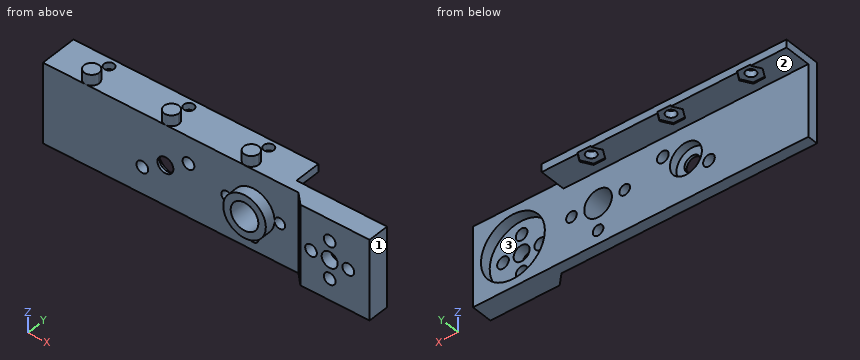
```python
from build123d import *

# Parameters (mm, degrees)
SKETCH_1_W          = 63
SKETCH_1_H          = 15
SKETCH_1_R          = 1.1
SKETCH_1_R_2        = 1
SKETCH_1_R_3        = 1.5
SKETCH_1_R_4        = 2.6
EXTRUDE_1_DEPTH     = 2
EXTRUDE_2_DEPTH     = 2
SKETCH_4_R          = 3
CUT_EXTRUDE_1_DEPTH = 1.5
SKETCH_5_W          = 46
SKETCH_5_H          = 1.5
EXTRUDE_3_DEPTH     = 5
SKETCH_2_3_R        = 0.95
CUT_EXTRUDE_2_DEPTH = 6
CUT_EXTRUDE_START   = -0.25
SKETCH_7_R          = 0.95
CUT_EXTRUDE_3_DEPTH = 0.25
SKETCH_1_3_W        = 15
SKETCH_1_3_H        = 15
SKETCH_1_3_R        = 6
SKETCH_1_3_R_2      = 1.5
SKETCH_1_3_R_3      = 1.1
EXTRUDE_4_DEPTH     = 2
EXTRUDE_START       = -2
SKETCH_1_4_W        = 15
SKETCH_1_4_H        = 15
SKETCH_1_4_R        = 6
SKETCH_1_4_R_2      = 1.5
SKETCH_1_4_R_3      = 1.1
EXTRUDE_5_DEPTH     = 2
SKETCH_1_5_R        = 6
CUT_EXTRUDE_4_DEPTH = 2
CUT_EXTRUDE_5_DEPTH = 15
SKETCH_1_6_R        = 4
SKETCH_1_6_R_2      = 2.6
EXTRUDE_6_DEPTH     = 2


with BuildPart() as part:
    # 草图1 → 凸台-拉伸1 (new body)
    with BuildSketch(Plane(origin=(0, 0, 0), x_dir=(1, 0, 0), z_dir=(0, 1, 0))):
        Rectangle(SKETCH_1_W, SKETCH_1_H)
        with Locations(Location((-4.169872981, -2.5, 0), (0, 0, 270))):
            Circle(SKETCH_1_R, mode=Mode.SUBTRACT)
        with Locations(Location((3, 0, 0), (0, 0, 270))):
            Circle(SKETCH_1_R_2, mode=Mode.SUBTRACT)
        with Locations(Location((13, 0, 0), (0, 0, 270))):
            Circle(SKETCH_1_R_2, mode=Mode.SUBTRACT)
        with Locations(Location((-8.5, 0, 0), (0, 0, 270))):
            Circle(SKETCH_1_R_3, mode=Mode.SUBTRACT)
        with Locations(Location((-12.830127019, 2.5, 0), (0, 0, 270))):
            Circle(SKETCH_1_R, mode=Mode.SUBTRACT)
        with Locations(Location((8, 5, 0), (0, 0, 270))):
            Circle(SKETCH_1_R_2, mode=Mode.SUBTRACT)
        with Locations(Location((8, 0, 0), (0, 0, 270))):
            Circle(SKETCH_1_R_4, mode=Mode.SUBTRACT)
        with Locations(Location((24, 3.5, 0), (0, 0, 270))):
            Circle(SKETCH_1_R, mode=Mode.SUBTRACT)
        with Locations(Location((24, -3.5, 0), (0, 0, 270))):
            Circle(SKETCH_1_R, mode=Mode.SUBTRACT)
        with Locations(Location((20.5, 0, 0), (0, 0, 270))):
            Circle(SKETCH_1_R, mode=Mode.SUBTRACT)
        with Locations(Location((24, 0, 0), (0, 0, 270))):
            Circle(SKETCH_1_R_3, mode=Mode.SUBTRACT)
        with Locations(Location((27.5, 0, 0), (0, 0, 270))):
            Circle(SKETCH_1_R, mode=Mode.SUBTRACT)
    extrude(amount=EXTRUDE_1_DEPTH)

    # 草图2 → 凸台-拉伸2 (add)
    with BuildSketch(Plane.XY.offset(7.5)):
        with BuildLine():
            Line((-22.1, 1.4), (-24.9, 1.4))
            ThreePointArc((-24.9, 1.4), (-23.5, 0), (-22.1, 1.4))
        make_face()
        with BuildLine():
            ThreePointArc((-24.764911064, 2), (-24.865810289, 1.707509764), (-24.9, 1.4))
            Line((-24.9, 1.4), (-22.1, 1.4))
            ThreePointArc((-22.1, 1.4), (-22.134189711, 1.707509764), (-22.235088936, 2))
            Line((-22.235088936, 2), (-24.764911064, 2))
        make_face()
        with BuildLine():
            ThreePointArc((-22.235088936, 2), (-23.5, 2.8), (-24.764911064, 2))
            Line((-24.764911064, 2), (-22.235088936, 2))
        make_face()
        with BuildLine():
            Line((-7.1, 1.4), (-9.9, 1.4))
            ThreePointArc((-9.9, 1.4), (-8.5, 0), (-7.1, 1.4))
        make_face()
        with BuildLine():
            ThreePointArc((-9.764911064, 2), (-9.865810289, 1.707509764), (-9.9, 1.4))
            Line((-9.9, 1.4), (-7.1, 1.4))
            ThreePointArc((-7.1, 1.4), (-7.134189711, 1.707509764), (-7.235088936, 2))
            Line((-7.235088936, 2), (-9.764911064, 2))
        make_face()
        with BuildLine():
            ThreePointArc((-7.235088936, 2), (-8.5, 2.8), (-9.764911064, 2))
            Line((-9.764911064, 2), (-7.235088936, 2))
        make_face()
        with BuildLine():
            Line((7.9, 1.4), (5.1, 1.4))
            ThreePointArc((5.1, 1.4), (6.5, 0), (7.9, 1.4))
        make_face()
        with BuildLine():
            ThreePointArc((5.235088936, 2), (5.134189711, 1.707509764), (5.1, 1.4))
            Line((5.1, 1.4), (7.9, 1.4))
            ThreePointArc((7.9, 1.4), (7.865810289, 1.707509764), (7.764911064, 2))
            Line((7.764911064, 2), (5.235088936, 2))
        make_face()
        with BuildLine():
            ThreePointArc((7.764911064, 2), (6.5, 2.8), (5.235088936, 2))
            Line((5.235088936, 2), (7.764911064, 2))
        make_face()
    extrude(amount=EXTRUDE_2_DEPTH)

    # 草图4 → 切除-拉伸1 (cut)
    with BuildSketch(Plane(origin=(0, 2, 0), x_dir=(1, 0, 0), z_dir=(0, 1, 0))):
        with Locations(Location((-8.5, 0, 0), (0, 0, 270))):
            Circle(SKETCH_4_R)
    extrude(amount=-CUT_EXTRUDE_1_DEPTH, mode=Mode.SUBTRACT)

    # 草图5 → 凸台-拉伸3 (add)
    with BuildSketch(Plane(origin=(0, 2, 0), x_dir=(1, 0, 0), z_dir=(0, 1, 0))):
        with Locations((-8.5, -6.75)):
            Rectangle(SKETCH_5_W, SKETCH_5_H)
    extrude(amount=EXTRUDE_3_DEPTH)

    # 草图2<3> → 切除-拉伸2 (cut)
    with BuildSketch(Plane.XY.offset(7.5)):
        with Locations((-23.5, 5.4)):
            Circle(SKETCH_2_3_R)
        with Locations((-8.5, 5.4)):
            Circle(SKETCH_2_3_R)
        with Locations((6.5, 5.4)):
            Circle(SKETCH_2_3_R)
    extrude(amount=-CUT_EXTRUDE_2_DEPTH, mode=Mode.SUBTRACT)

    # 草图7 → 切除-拉伸3 (cut)
    # profile 1 of 3: a face of its own
    with BuildSketch(Plane(origin=(0, 0, 6), x_dir=(-1, 0, 0), z_dir=(0, 0, -1)).offset(CUT_EXTRUDE_START)):
        Polygon((-7.596965511, 3.5), (-5.403034489, 3.5), (-4.306068977, 5.4), (-5.403034489, 7.3), (-7.596965511, 7.3), (-8.693931023, 5.4), align=None)
        with Locations(Location((-6.5, 5.4, 0), (0, 0, 180))):
            Circle(SKETCH_7_R, mode=Mode.SUBTRACT)
    # profile 2 of 3: a face of its own
    with BuildSketch(Plane(origin=(0, 0, 6), x_dir=(-1, 0, 0), z_dir=(0, 0, -1)).offset(CUT_EXTRUDE_START)):
        Polygon((6.306068977, 5.4), (7.403034489, 3.5), (9.596965511, 3.5), (10.693931023, 5.4), (9.596965511, 7.3), (7.403034489, 7.3), align=None)
        with Locations(Location((8.5, 5.4, 0), (0, 0, 180))):
            Circle(SKETCH_7_R, mode=Mode.SUBTRACT)
    # profile 3 of 3: a face of its own
    with BuildSketch(Plane(origin=(0, 0, 6), x_dir=(-1, 0, 0), z_dir=(0, 0, -1)).offset(CUT_EXTRUDE_START)):
        Polygon((21.306068977, 5.4), (22.403034489, 3.5), (24.596965511, 3.5), (25.693931023, 5.4), (24.596965511, 7.3), (22.403034489, 7.3), align=None)
    extrude(amount=CUT_EXTRUDE_3_DEPTH, mode=Mode.SUBTRACT)

    # 草图1<3> → 凸台-拉伸4 (add)
    # profile 1 of 2: a face of its own
    with BuildSketch(Plane(origin=(0, 0, 0), x_dir=(1, 0, 0), z_dir=(0, 1, 0))):
        with Locations((24, 0)):
            Rectangle(SKETCH_1_3_W, SKETCH_1_3_H)
        with Locations((24, 0)):
            Circle(SKETCH_1_3_R, mode=Mode.SUBTRACT)
    # profile 2 of 2: a face of its own
    with BuildSketch(Plane(origin=(0, 0, 0), x_dir=(1, 0, 0), z_dir=(0, 1, 0))):
        with Locations((24, 0)):
            Circle(SKETCH_1_3_R)
        with Locations(Location((24, 0, 0), (0, 0, 270))):
            Circle(SKETCH_1_3_R_2, mode=Mode.SUBTRACT)
        with Locations(Location((27.5, 0, 0), (0, 0, 270))):
            Circle(SKETCH_1_3_R_3, mode=Mode.SUBTRACT)
        with Locations(Location((24, -3.5, 0), (0, 0, 270))):
            Circle(SKETCH_1_3_R_3, mode=Mode.SUBTRACT)
        with Locations(Location((20.5, 0, 0), (0, 0, 270))):
            Circle(SKETCH_1_3_R_3, mode=Mode.SUBTRACT)
        with Locations(Location((24, 3.5, 0), (0, 0, 270))):
            Circle(SKETCH_1_3_R_3, mode=Mode.SUBTRACT)
    extrude(amount=EXTRUDE_4_DEPTH)

    # 草图1<4> → 凸台-拉伸5 (add)
    # profile 1 of 2: a face of its own
    with BuildSketch(Plane(origin=(0, 0, 0), x_dir=(1, 0, 0), z_dir=(0, 1, 0)).offset(EXTRUDE_START)):
        with Locations((24, 0)):
            Rectangle(SKETCH_1_4_W, SKETCH_1_4_H)
        with Locations((24, 0)):
            Circle(SKETCH_1_4_R, mode=Mode.SUBTRACT)
    # profile 2 of 2: a face of its own
    with BuildSketch(Plane(origin=(0, 0, 0), x_dir=(1, 0, 0), z_dir=(0, 1, 0)).offset(EXTRUDE_START)):
        with Locations((24, 0)):
            Circle(SKETCH_1_4_R)
        with Locations(Location((24, 0, 0), (0, 0, 270))):
            Circle(SKETCH_1_4_R_2, mode=Mode.SUBTRACT)
        with Locations(Location((27.5, 0, 0), (0, 0, 270))):
            Circle(SKETCH_1_4_R_3, mode=Mode.SUBTRACT)
        with Locations(Location((24, -3.5, 0), (0, 0, 270))):
            Circle(SKETCH_1_4_R_3, mode=Mode.SUBTRACT)
        with Locations(Location((20.5, 0, 0), (0, 0, 270))):
            Circle(SKETCH_1_4_R_3, mode=Mode.SUBTRACT)
        with Locations(Location((24, 3.5, 0), (0, 0, 270))):
            Circle(SKETCH_1_4_R_3, mode=Mode.SUBTRACT)
    extrude(amount=EXTRUDE_5_DEPTH)

    # 草图1<5> → 切除-拉伸4 (cut)
    with BuildSketch(Plane(origin=(0, 0, 0), x_dir=(1, 0, 0), z_dir=(0, 1, 0))):
        with Locations(Location((24, 0, 0), (0, 0, 270))):
            Circle(SKETCH_1_5_R)
    extrude(amount=CUT_EXTRUDE_4_DEPTH, mode=Mode.SUBTRACT)

    # 草图8 → 切除-拉伸5 (cut)
    with BuildSketch(Plane(origin=(0, 0, -7.5), x_dir=(-1, 0, 0), z_dir=(0, 0, -1))):
        Polygon((-16.5, 0), (-18.5, -2), (-16.5, -2), align=None)
    extrude(amount=-CUT_EXTRUDE_5_DEPTH, mode=Mode.SUBTRACT)

    # 草图1<6> → 凸台-拉伸6 (add)
    with BuildSketch(Plane(origin=(0, 0, 0), x_dir=(1, 0, 0), z_dir=(0, 1, 0)).offset(EXTRUDE_START)):
        with Locations(Location((8, 0, 0), (0, 0, 270))):
            Circle(SKETCH_1_6_R)
        with Locations(Location((8, 0, 0), (0, 0, 270))):
            Circle(SKETCH_1_6_R_2, mode=Mode.SUBTRACT)
    extrude(amount=EXTRUDE_6_DEPTH)


solid = part.part
```
Could you check a few things on this model? Use its own coordinates, in mm. Face numbers are marked on the shaded views. Round coordinates to 2 decimals unless told otherwise and drop trailing zeros. Write each loop counter-clockwise with the first axis right and the second up, starting at its lowest first coordinate (ties: lowest second). Pieces come first, ordered by that corner, then holes.
(1) If I drill on probe 1 along X at (y, z) = (-0.7, 0); probe 2 along X at (y, z) = (-0.25, -3.25); probe 3 along X at (y, z) = (1, 5.5), over which ranges is the centre line in solid material (lowest first)?
Findings below:
probe 1: x = 4 to 5.4, 10.6 to 12, 17.2 to 19.4, 21.6 to 22.5, 25.5 to 26.4, 28.6 to 31.5
probe 2: x = 5.67 to 10.33, 16.75 to 22.93, 25.07 to 31.5
probe 3: x = -31.5 to 21.6, 26.4 to 31.5
(2) Suppose I cut it at A-A on y = -0.75. Write out the boundary of the cut face in (x, z).
Findings below:
outline: circle Ø8 at (8, 0); (17.25, -7.5) - (31.5, -7.5) - (31.5, 7.5) - (17.25, 7.5) - close; hole circle Ø5.2 at (8, 0); hole circle Ø2.2 at (20.5, 0); hole circle Ø3 at (24, 0); hole circle Ø2.2 at (24, -3.5); hole circle Ø2.2 at (24, 3.5); hole circle Ø2.2 at (27.5, 0)
(3) Suppose I cut it at C-C on x = -2.5. Write out the boundary of the cut face in (y, z).
Findings below:
outline: (0, -7.5) - (2, -7.5) - (2, 6) - (7, 6) - (7, 7.5) - (0, 7.5) - close
(4) Thinking about a two-plate mould opening in X: for the marked faces 1, 2 and 3, which applies, +X half, -X half, draft (parallel to the pull), parting line (faces both ways), or undercut?
Findings below:
face 1: +X half
face 2: draft
face 3: undercut
(5) For pin 1 (1 mm diameter, centred on x = 2, z = -3, fed in from +Y); pin 2 (9.5 mm diameter, centred on x = 24, z = 0, fed in from +Y); pin 3 (1.8 mm diameter, centred on x = 24, z = -3.5, fed in from +Y); pin 4 (4 mm diameter, centred on x = -23.5, y = 3, fed in from -Z), each with a flat end and sliding along its axis, tell me the tip position at first contact or that it passes through.
Findings below:
pin 1: stops at y = 2
pin 2: stops at y = 0
pin 3: passes through
pin 4: stops at z = -7.5
(6) Suppose I cut it at B-B on x = 24. Write out the boundary of the cut face in (y, z).
Findings below:
outline: (-2, -7.5) - (2, -7.5) - (2, -6) - (0, -6) - (0, -4.6) - (-2, -4.6) - close; (-2, -2.4) - (0, -2.4) - (0, -1.5) - (-2, -1.5) - close; (-2, 1.5) - (0, 1.5) - (0, 2.4) - (-2, 2.4) - close; (-2, 4.6) - (0, 4.6) - (0, 6) - (2, 6) - (2, 7.5) - (-2, 7.5) - close
